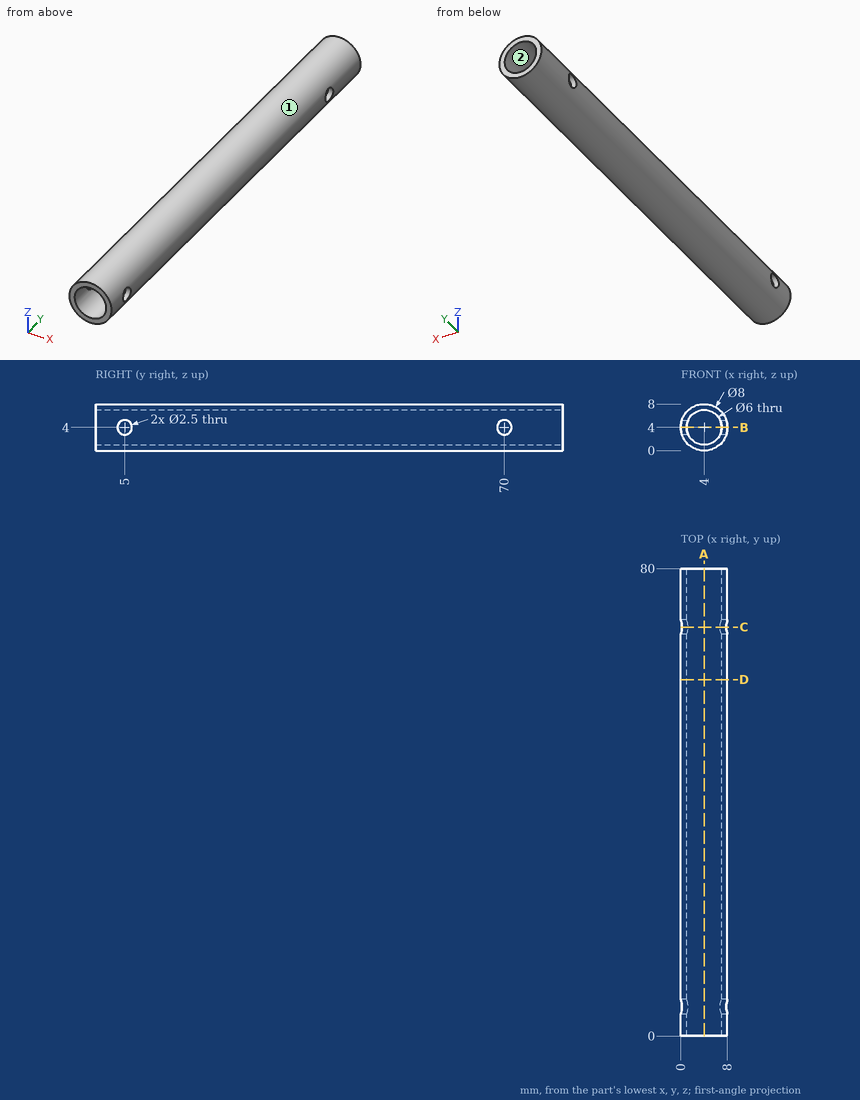
Part print with two shaded views. Sizes in mm from the minimum x, y, z corner. Coordinates: 2 decimals unless noted, no trailing zeros. Write each loop counter-clockwise with the first axis right and the second up, starting at its lowest first coordinate (ties: lowest second). Pieces come first, ordered by that corner, then holes.
1. Drill centre lines: probe 1 along Y at (x, z) = (7.35, 4); probe 2 along X at (y, z) = (46.5, 4); probe 3 along Z at (x, y) = (5.25, 36). Where is each one in solid material? Low to high.
Answer block:
probe 1: y = 0 to 3.75, 6.25 to 68.75, 71.25 to 80
probe 2: x = 0 to 1, 7 to 8
probe 3: z = 0.2 to 1.27, 6.73 to 7.8
2. Drop flat-ended pins along their axis: pin 1 (2 mm diameter, centred on y = 5, z = 4, fed in from +X); pin 2 (2 mm diameter, centred on y = 13, z = 1, fed in from +X). Give the stop position or say it passes through.
Answer block:
pin 1: passes through
pin 2: stops at x = 7.46
3. Band-saw the part on B-B, the plane z = 4. Give the cut face in (x, y), and give its area (3 significant figures).
Answer block:
outline: (0, 0) - (1, 0) - (1, 3.75) - (0, 3.75) - close; (0, 6.25) - (1, 6.25) - (1, 68.75) - (0, 68.75) - close; (0, 71.25) - (1, 71.25) - (1, 80) - (0, 80) - close; (7, 0) - (8, 0) - (8, 3.75) - (7, 3.75) - close; (7, 6.25) - (8, 6.25) - (8, 68.75) - (7, 68.75) - close; (7, 71.25) - (8, 71.25) - (8, 80) - (7, 80) - close
area: 150 mm2
4. Pull direction X, two halves, no side cores. Call the marked faces 1 and 2: released by +X, released by -X, zero draft, split by the parting line, or undercut.
Answer block:
face 1: split by the parting line
face 2: undercut
5. Band-saw the part on D-D, the plane y = 61. Give the cut face in (x, z).
Answer block:
outline: circle Ø8 at (4, 4); hole circle Ø6 at (4, 4)
6. Band-saw the part on A-A, the plane x = 4. Give the cut face in (y, z), and give its area (3 significant figures).
Answer block:
outline: (0, 0) - (80, 0) - (80, 1) - (0, 1) - close; (0, 7) - (80, 7) - (80, 8) - (0, 8) - close
area: 160 mm2
7. Band-saw the part on C-C, the plane y = 70. Give the cut face in (x, z), and give its area (3 significant figures).
Answer block:
outline: (0.2, 2.75) arc R4 ccw to (7.8, 2.75) - (6.73, 2.75) arc R3 cw to (1.27, 2.75) - close; (0.2, 5.25) - (1.27, 5.25) arc R3 cw to (6.73, 5.25) - (7.8, 5.25) arc R4 ccw to start
area: 16.9 mm2
